Could you check a few things on this model? Use its own coordinates, in mm. A direction names the side the tool comes from. Give positions to 0.01 mm unless a question says otherwise; leave off trailing zeros. Write each loop counter-clockwise with the first axis right and the second up, starting at its lowest first coordinate (ties: lowest second). Pieces come first, ordered by that corner, then holes. Notation, with made-up numbers: (-32.75, 10) -> (-25.75, 10) arc R15 ccw to (-25.75, 37) -> close; hole circle Ø9 at (34, -30.75). An arc over 180 degrees is marked (long way). Write item = value, one per line. Start each with the question number.
```python
from build123d import *

# Parameters (mm, degrees)
F1_DEPTH = 10
F2_R     = 1.5
F3_DEPTH = 10.5
F4_R     = 1.5
F5_DEPTH = 25
F6_DEPTH = 2
F7_SIZE  = 2
F8_SIZE  = 2
F9_R     = 2


with BuildPart() as f1:
    # F0 (on Front) → F1 (new body)
    with BuildSketch(Plane.XZ):
        Polygon((-20, -11.5), (20, -11.5), (20, -6.5), (9, -6.5), (9, 11.5), (0.5, 11.5), (0.5, 6.5086536296), (5, 6.5086536296), (5, -3.4913463704), (-5, -3.4913463704), (-5, 6.5086536296), (-0.5, 6.5086536296), (-0.5, 11.5), (-9, 11.5), (-9, -6.5), (-20, -6.5), align=None)
    extrude(amount=F1_DEPTH)

    # F2 (on face) → F3 (cut)
    with BuildSketch(Plane(origin=(0, 0, -11.5), x_dir=(1, 0, 0), z_dir=(0, 0, -1))):
        with Locations((16, 4.8524653539)):
            Circle(F2_R)
        with Locations((-16, 4.8524653539)):
            Circle(F2_R)
    extrude(amount=-F3_DEPTH, mode=Mode.SUBTRACT)

    # F4 (on face) → F5 (cut)
    with BuildSketch(Plane(origin=(-9, 0, 0), x_dir=(0, -1, 0), z_dir=(-1, 0, 0))):
        with Locations((5, 9.5)):
            Circle(F4_R)
    extrude(amount=-F5_DEPTH, mode=Mode.SUBTRACT)

    # F6 (add): faces of the model
    f6_faces = [f1.faces().sort_by_distance(p)[0] for p in [
        (4.75, -5, 11.5),
        (-4.75, -5, 11.5),
    ]]
    extrude(f6_faces, amount=F6_DEPTH)

    # F7
    f7_edges = [f1.edges().sort_by_distance(p)[0] for p in [
        (-9, -5, -6.5),
    ]]
    chamfer(f7_edges, length=F7_SIZE)

    # F8
    f8_edges = [f1.edges().sort_by_distance(p)[0] for p in [
        (9, -5, -6.5),
    ]]
    chamfer(f8_edges, length=F8_SIZE)

    # F9
    f9_edges = [f1.edges().sort_by_distance(p)[0] for p in [
        (-20, -10, -9),
        (-20, 0, -9),
        (20, 0, -9),
        (20, -10, -9),
        (9, -5, 13.5),
        (-9, -5, 13.5),
        (-9, -10, 4.5),
        (9, -10, 4.5),
        (9, 0, 4.5),
        (-9, 0, 4.5),
        (0, 0, -11.5),
        (0, -10, -11.5),
    ]]
    fillet(f9_edges, radius=F9_R)


solid = f1.part
```
(1) On a 3-axis mill with a long thin cutter (end or side, diameter ignored), from which of +Z, -Z, +X, -X, +Y, -Y can I reach the whole of each face in a straight line? I mean faces 4 (the flat face through (14.6, -3.8, -6.5)), 5 (the flat face through (-5, -5, 1)), 6 (the flat face through (0.5, -6, 11)). Say none if no direction works.
(2) If I drill on line 1 along Z through (x, y) = (3.5, -8); line 2 along Z through (x, y) = (-6.75, -5); line 3 along Z through (x, y) = (-4, -5), over which ranges is the centre line in solid material (lowest first)? Write a range as from..to.
(3) Imagine slicing it at B-B (x = 16). Please give me the cut outline in (y, z), then the cut area to 3 significant figures.
(4) I'm going to push flat-ended pins straight in: pin 1 (3.5 mm diameter, centred on y = -5, z = 9.5, fed in from -X); pin 2 (1.8 mm diameter, centred on y = -5, z = 4.5, fed in from +X); pin 3 (3.5 mm diameter, centred on x = 16, y = -4.85, fed in from +Z); pin 4 (4 mm diameter, centred on x = -12.5, z = -3, fed in from -Y). Where does each tip first touch, or does it pass through?
(5) Imagine slicing it at D-D (x = -6). Please give me the cut outline in (y, z), then the cut area to 3 significant figures.
(6) Imagine slicing it at C-C (z = 7). Please give me the cut outline in (x, y), then the cut area to 3 significant figures.
(7) We'd pull the mould along Y, two halves only. Please class faces 1 (the flat face through (-9, -5, 4)), 2 (the cylindrical face through (-8.43, -9.4, 4.37)), 3 (the cylindrical face through (-17.5, -4.9, -9)): released by +Y, released by -Y, zero draft, split by the parting line, or undercut.
(8) Imagine slicing it at A-A (z = 9.5). Please give me the cut outline in (x, y), then the cut area to 3 significant figures.
Answers below:
q1.face_4 = +Z, +X, +Y, -Y
q1.face_5 = +Y, -Y
q1.face_6 = +Z, +Y, -Y
q2.line_1 = -11.5..-3.49, 6.51..13.5
q2.line_2 = -11.5..8, 11..13.5
q2.line_3 = -11.5..-3.49, 6.51..8, 11..13.5
q3.outline = (-10, -9.5) arc R2 ccw to (-8, -11.5) -> (-6.35, -11.5) -> (-6.35, -6.5) -> (-10, -6.5) -> close; (-3.35, -11.5) -> (-2, -11.5) arc R2 ccw to (0, -9.5) -> (0, -6.5) -> (-3.35, -6.5) -> close
q3.area = 33.3 mm^2
q4.pin_1 = -9
q4.pin_2 = 9
q4.pin_3 = -6.5
q4.pin_4 = through
q5.outline = (-10, -9.5) arc R2 ccw to (-8, -11.5) -> (-2, -11.5) arc R2 ccw to (0, -9.5) -> (0, 13.5) -> (-10, 13.5) -> close; hole circle Ø3 at (-5, 9.5)
q5.area = 241 mm^2
q6.outline = (-9, -8) arc R2 ccw to (-7, -10) -> (-0.5, -10) -> (-0.5, 0) -> (-7, 0) arc R2 ccw to (-9, -2) -> close; (0.5, -10) -> (7, -10) arc R2 ccw to (9, -8) -> (9, -2) arc R2 ccw to (7, 0) -> (0.5, 0) -> close
q6.area = 167 mm^2
q7.face_1 = zero draft
q7.face_2 = released by -Y
q7.face_3 = undercut
q8.outline = (-9, -8) arc R2 ccw to (-7, -10) -> (-0.5, -10) -> (-0.5, -6.5) -> (-9, -6.5) -> close; (-9, -3.5) -> (-0.5, -3.5) -> (-0.5, 0) -> (-7, 0) arc R2 ccw to (-9, -2) -> close; (0.5, -10) -> (7, -10) arc R2 ccw to (9, -8) -> (9, -6.5) -> (0.5, -6.5) -> close; (0.5, -3.5) -> (9, -3.5) -> (9, -2) arc R2 ccw to (7, 0) -> (0.5, 0) -> close
q8.area = 116 mm^2
